Geometry check sheet. Reference: drawing and pictorial views, mm from the part's lowest x, y, z. A direction names the side the tool comes from. Give positions to 0.01 mm unless a question says otherwise; leave off trailing zeros. Order: outer loops, then holes, each group sorted by start corner. A loop starts at its lowest first (then second) coordinate and runs counter-clockwise, first axis right, second up. Notation, with made-up numbers: (-10, 23.5) -> (16, 23.5) arc R21 ccw to (16, 61.5) -> close; hole circle Ø9 at (-9, 79.25). An arc over 180 degrees is marked (long way). Write each question's results on one line, items separated by ' | '. Start each with the question number.
1. Mould release check, pull along X, two halves, no side actions. Record for the marked faces 4, 5 and 6: +X half, -X half, draft (parallel to the pull), parting line (faces both ways), or undercut.
2. Cross-section at B-B, the plane y = 1.3. Enter the section's corners in (x, z) (1 decimal), then the cut area to 3 significant figures.
3. Material ranges on L1, parallel to X at y = 2.4, z = 13.25 (1 decimal); L2, parallel to X at y = 0.85, z = 11; L3, parallel to Z at x = 11.75, y = 3.25 (1 decimal), recorded low to high. Write a range as from..to.
4. Depth check by flat-ended pin: pin 1 Ø2 at (y, z) = (1, 8) entering from +X. Enter the tip coordinate at first touch or a pass-through.
5. Set-up check for the marked faces 1, 2 and 3: record each of +Z, -Z, +X, -X, +Y, -Y from which the full face is reachable in a straight line by a thin tool's end or side.
6. Cross-section at A-A, the plane z = 12. Enter the section's corners in (x, y).
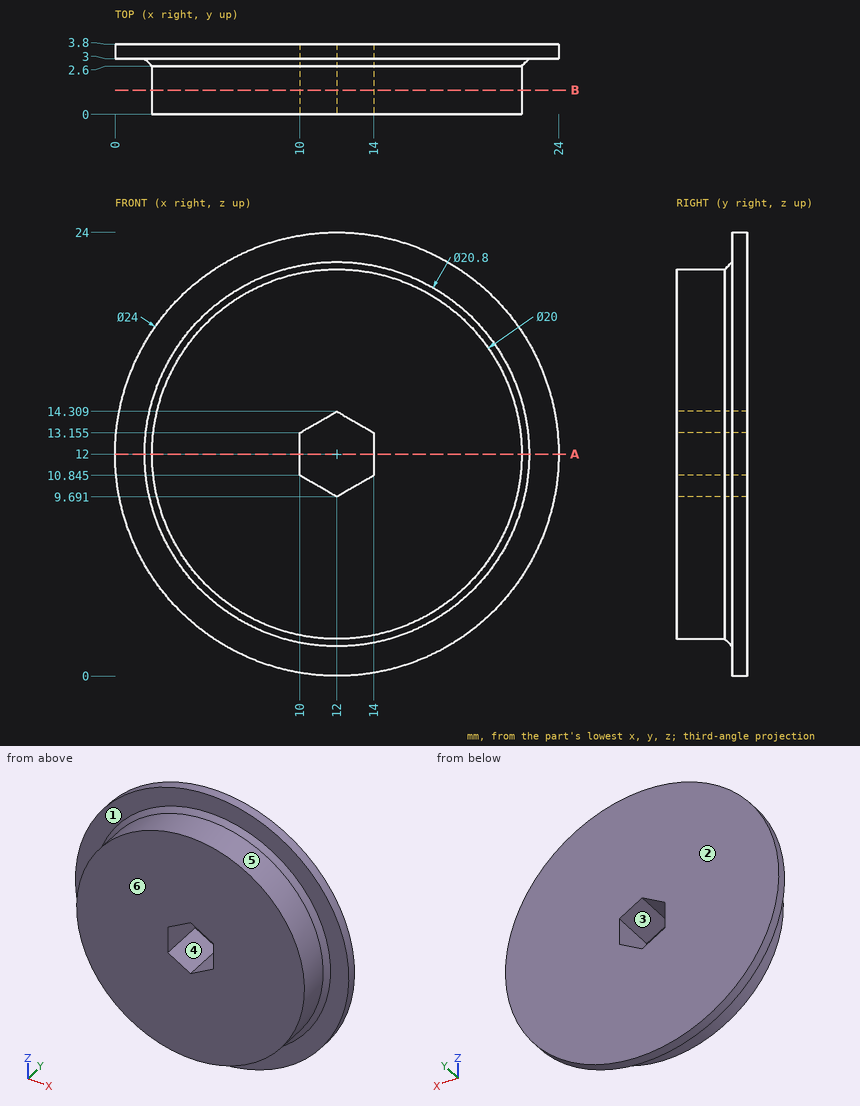
Results below:
1) face 4: undercut | face 5: parting line | face 6: draft
2) outline: circle Ø20 at (12, 12); hole (10, 10.8) -> (12, 9.7) -> (14, 10.8) -> (14, 13.2) -> (12, 14.3) -> (10, 13.2) -> close | area: 300 mm²
3) L1: x = 2.1..10.2, 13.8..21.9 | L2: x = 2.05..10, 14..21.95 | L3: z = 0..9.8, 14.2..24
4) pin 1: stops at x = 21.54
5) face 1: -Y | face 2: +Z, -Z, +X, -X, +Y | face 3: +Y, -Y
6) outline: (0, 3) -> (1.6, 3) -> (2, 2.6) -> (2, 0) -> (10, 0) -> (10, 3.8) -> (0, 3.8) -> close; (14, 0) -> (22, 0) -> (22, 2.6) -> (22.4, 3) -> (24, 3) -> (24, 3.8) -> (14, 3.8) -> close
